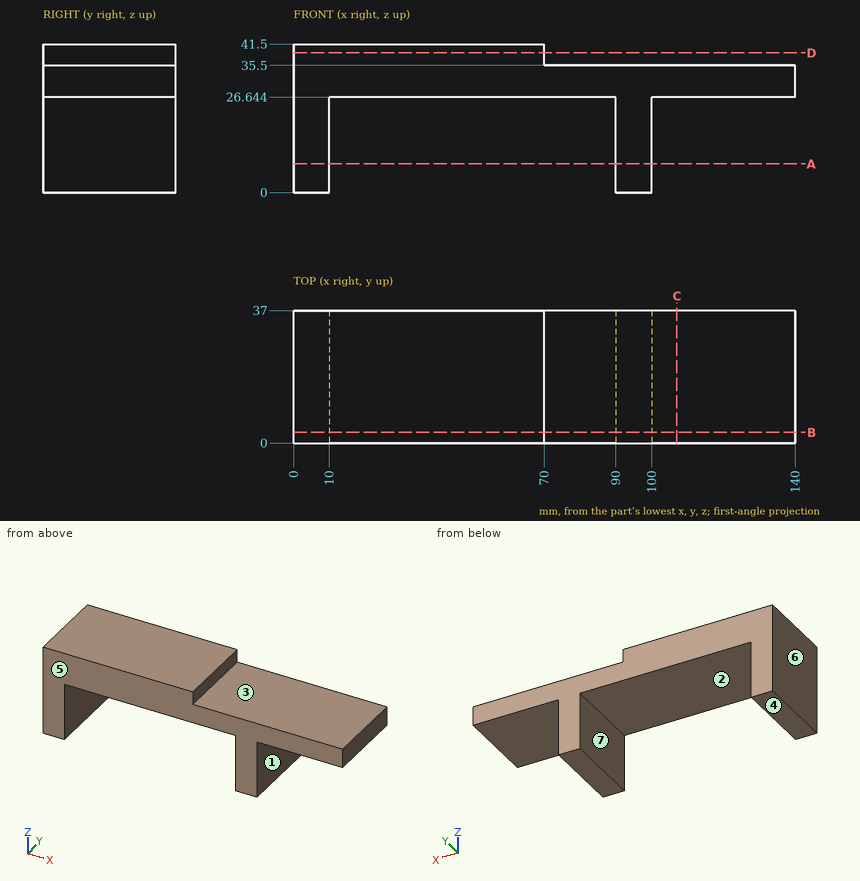
Input: dimensioned drawing with shaded views. Units: mm. Origin: part minimum x, y, z. A direction names the side the tool comes from. Coordinates: 2 decimals unless noted, no trailing zeros. Loops run counter-clockwise (first coordinate to the right, second up) from the corner with the lowest first, then second, coordinate; pieces in that order, holes last. Notation, with made-up numbers: M -34,13 L 12,13 A31 cw 12,45 Z; hole C 7,60.5 d9. An arc over 180 degrees is marked long. Put each result on its own line as item: value.
(1) First-contact query: pin 1 (4 mm diameter, centred on y = 12.5, z = 11.5, fed in from -X); pin 2 (6 mm diameter, centred on x = 64.5, z = 22, fed in from -Y); pin 3 (8 mm diameter, centred on y = 27.5, z = 18.5, fed in from +X); pin 4 (2 mm diameter, centred on x = 90.5, y = 10.5, fed in from +Z). Flat tips, straight axial feed; report the tip coordinate or a pass-through.
Answer sheet:
pin 1: stops at x = 0
pin 2: passes through
pin 3: stops at x = 100
pin 4: stops at z = 35.5
(2) Access query for the marked faces 1, 2, 3 and 4. Directions: +Z, -Z, +X, -X, +Y, -Y. A direction counts if a zero-diameter tool reaches every point of the face in a straight line with its end or side. Return the directions, or none.
Answer sheet:
face 1: -Z, +X, +Y, -Y
face 2: -Z, +Y, -Y
face 3: +Z, +X, +Y, -Y
face 4: -Z, +X, -X, +Y, -Y
(3) Cut plane A-A on z = 8. Return the cut outline in (x, y).
Answer sheet:
outline: M 0,0 L 10,0 L 10,37 L 0,37 Z; M 90,0 L 100,0 L 100,37 L 90,37 Z
(4) Cut plane D-D on z = 39. Return the cut outline in (x, y), then the cut area to 3 significant figures.
Answer sheet:
outline: M 0,0 L 70,0 L 70,37 L 0,37 Z
area: 2,590 mm^2
(5) Material intervals for probe 1 along X at (y, z) = (3, 24.5); probe 2 along X at (y, z) = (17.5, 37.5); probe 3 along Z at (x, y) = (80, 22), sorted ascending.
Answer sheet:
probe 1: x = 0 to 10, 90 to 100
probe 2: x = 0 to 70
probe 3: z = 26.64 to 35.5
(6) Cut plane C-C on x = 107. Return the cut outline in (y, z), then the cut area to 3 significant figures.
Answer sheet:
outline: M 0,26.64 L 37,26.64 L 37,35.5 L 0,35.5 Z
area: 328 mm^2
(7) Cut plane B-B on y = 3. Return the cut outline in (x, z).
Answer sheet:
outline: M 0,0 L 10,0 L 10,26.64 L 90,26.64 L 90,0 L 100,0 L 100,26.64 L 140,26.64 L 140,35.5 L 70,35.5 L 70,41.5 L 0,41.5 Z
(8) Draft query along X for the marked faces 5, 6 and 7. Return one class per face: pulls with the +X half, pulls with the -X half, needs draft (parallel to the pull), parting line crosses it, or undercut.
Answer sheet:
face 5: needs draft
face 6: pulls with the -X half
face 7: undercut
